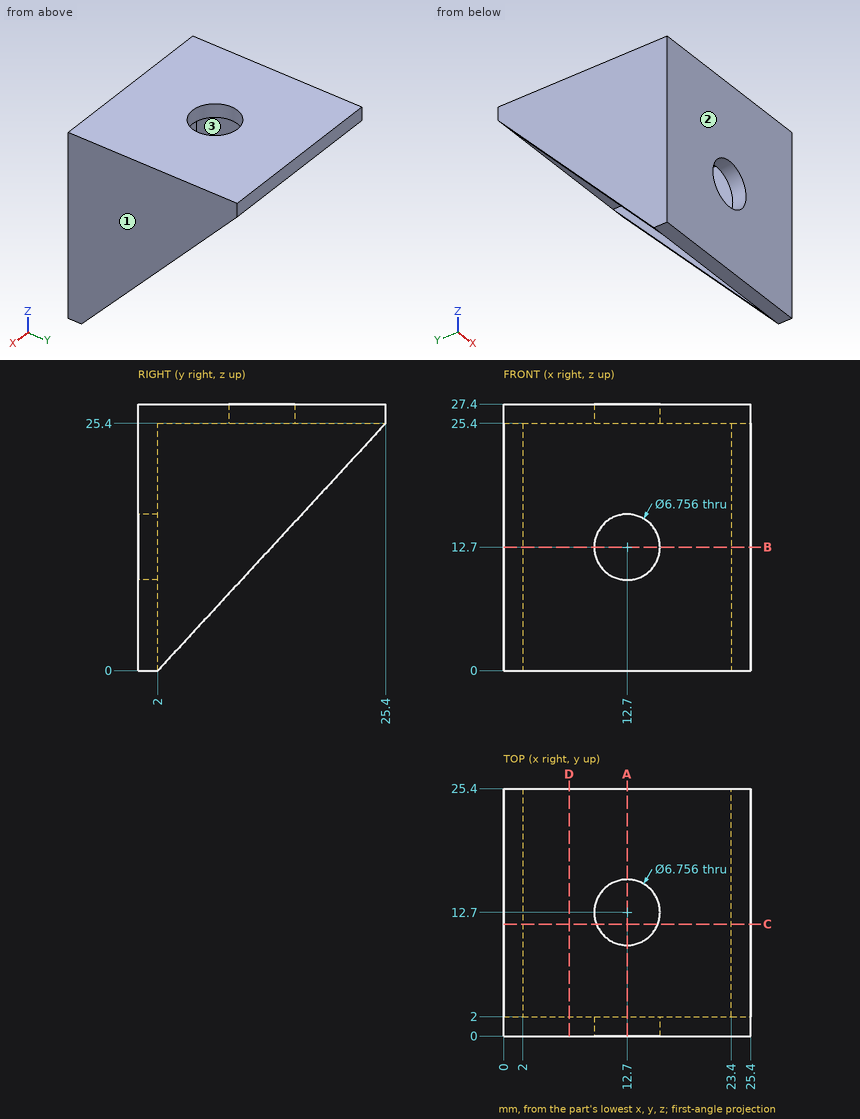
For this review, use the dimensioned drawing (mm, ordinates from the lowest corner) and the shaded views. Coordinates: 2 decimals unless noted, no trailing zeros. Loops run counter-clockwise (first coordinate to the right, second up) from the corner with the lowest first, then second, coordinate; pieces in that order, holes last. Notation, with made-up numbers: (55, 42.5) - (64, 42.5) arc R23 cw to (64, 57.5) - close; hole circle Ø3 at (1.25, 44.5). An arc over 180 degrees is marked (long way). Use one line per item in the form item = value. Start each with the question number.
1) For pin 1 (10.5 mm diameter, centred on x = 9.5, y = 13.5, fed in from -Z); pin 2 (8 mm diameter, centred on x = 12.7, z = 12.7, fed in from +Y), all flat-tipped, find the tip position at first contact; note any pin that passes through.
2) Take a section at D-D (x = 6.75). State the section outline as (y, z) points.
3) To check wall thickness, follow probe 1 along X at (y, z) = (2.75, 6.75); probe 2 along Z at (x, y) = (12.7, 1.5); probe 3 along Y at (x, z) = (12.7, 26.95). State the ranges of each line that lie inside material, in increasing order. Write a range as from..to.
4) Take a section at C-C (y = 11.5). State the section outline as (x, z) points.
5) Take a section at A-A (x = 12.7). State the section outline as (y, z) points.
6) Draft analysis for pull direction X (two halves, no side actions). For the marked faces 1, 2 and 3, state which applies: released by +X, released by -X, zero draft, split by the parting line, or undercut.
7) Take a section at B-B (z = 12.7). State the section outline as (x, y) points.
From the geometry:
q1.pin_1 = 25.4
q1.pin_2 = 2
q2.outline = (0, 0) - (2, 0) - (2, 25.4) - (25.4, 25.4) - (25.4, 27.4) - (0, 27.4) - close
q3.probe_1 = 0..2, 23.4..25.4
q3.probe_2 = 0..9.32, 16.08..27.4
q3.probe_3 = 0..9.32, 16.08..25.4
q4.outline = (0, 10.31) - (2, 10.31) - (2, 25.4) - (9.54, 25.4) - (9.54, 27.4) - (0, 27.4) - close; (15.86, 25.4) - (23.4, 25.4) - (23.4, 10.31) - (25.4, 10.31) - (25.4, 27.4) - (15.86, 27.4) - close
q5.outline = (0, 0) - (2, 0) - (2, 9.32) - (0, 9.32) - close; (0, 16.08) - (2, 16.08) - (2, 25.4) - (9.32, 25.4) - (9.32, 27.4) - (0, 27.4) - close; (16.08, 25.4) - (25.4, 25.4) - (25.4, 27.4) - (16.08, 27.4) - close
q6.face_1 = released by +X
q6.face_2 = zero draft
q6.face_3 = undercut
q7.outline = (0, 0) - (9.32, 0) - (9.32, 2) - (2, 2) - (2, 13.7) - (0, 13.7) - close; (16.08, 0) - (25.4, 0) - (25.4, 13.7) - (23.4, 13.7) - (23.4, 2) - (16.08, 2) - close
